```python
from build123d import *

# Parameters (mm, degrees)
SKETCH1_R                = 5
BOSS_EXTRUDE1_DEPTH      = 28
BOSS_EXTRUDE1_DEPTH_BACK = 28
SKETCH2_R                = 14.7
SKETCH2_R_2              = 4.7
CUT_EXTRUDE_THIN1_DEPTH  = 0.7
CHAMFER1_SIZE            = 1


with BuildPart() as part:
    # Sketch1 → Boss-Extrude1 (new body, two sides)
    with BuildSketch(Plane.XY) as boss_extrude1_sk:
        Circle(SKETCH1_R)
    extrude(amount=BOSS_EXTRUDE1_DEPTH)
    extrude(boss_extrude1_sk.sketch, amount=-BOSS_EXTRUDE1_DEPTH_BACK)

    # Sketch2 → Cut-Extrude-Thin1 (cut)
    with BuildSketch(Plane.XY.offset(25)):
        Circle(SKETCH2_R)
        Circle(SKETCH2_R_2, mode=Mode.SUBTRACT)
    cut_extrude_thin1 = extrude(amount=CUT_EXTRUDE_THIN1_DEPTH, mode=Mode.SUBTRACT)

    # Mirror1: Cut-Extrude-Thin1 across plane
    add(cut_extrude_thin1.mirror(Plane.XY), mode=Mode.SUBTRACT)

    # Chamfer1
    chamfer1_edges = [part.edges().sort_by_distance(p)[0] for p in [
        (-5, 0, -28),
        (-5, 0, 28),
    ]]
    chamfer(chamfer1_edges, length=CHAMFER1_SIZE)


solid = part.part
```
The listing builds one solid part. Answer for the finished solid, in the listing's coordinates (mm). Coordinates: 2 decimals unless noted, no trailing zeros. Write each loop counter-clockwise with the first axis right and the second up, starting at its lowest first coordinate (ties: lowest second). Pieces come first, ordered by that corner, then holes. Notation, with made-up numbers: (79.5, 0) - (116.5, 0) arc R15 ccw to (116.5, 4) - close; hole circle Ø11 at (-22.75, 44.25). An arc over 180 degrees is marked (long way). Return JSON: item names as keys, results as strings. Group by question number.
1. Straight lines are drawn through the part: L1, parallel to Z at x = -3, y = 3.75; L2, parallel to Y at x = -0.25, z = -26; L3, parallel to X at y = -3, z = 16.5. For each, find the intervals that lie inside material, in ascending order.
2. Given pin 1 (5 mm diameter, centred on y = 3.5, z = -18, fed in from -X); pin 2 (4 mm diameter, centred on x = 3, z = -11, fed in from +Y); pin 3 (4 mm diameter, centred on y = 3, z = -12, fed in from +X), each flat-ended and moving along its own axis, determine where each tip first touches the part or whether it passes through.
3. A cutting plane is placed at A-A, the plane z = 5. Determine the outline of the cut face in (x, y).
4. Determine the mould class of faces 1 (the cylindrical face through (-1.02, -4.59, -25.35)), 2 (the cylindrical face through (-1.08, -4.88, 0.35)), 3 (the flat face through (0, 0, -28)), 4 (the cylindrical face through (-1.02, -4.59, 25.35)) for opening direction Z: released by +Z, released by -Z, zero draft, split by the parting line, or undercut.
Ans:
{
 "1": {"L1": "-27.2 to -25.7, -25 to 25, 25.7 to 27.2", "L2": "-4.99 to 4.99", "L3": "-4 to 4"},
 "2": {"pin 1": "x = -4.9", "pin 2": "y = 4.9", "pin 3": "x = 4.9"},
 "3": {"outline": "circle Ø10 at (0, 0)"},
 "4": {"face 1": "undercut", "face 2": "zero draft", "face 3": "released by -Z", "face 4": "undercut"}
}
